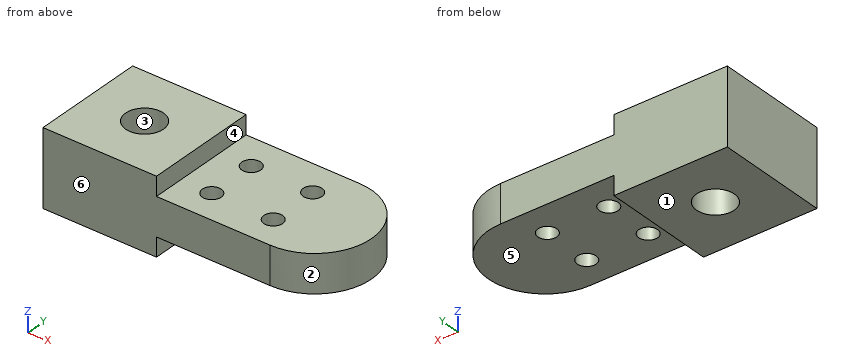
from build123d import *

# Parameters (mm, degrees)
F0_W     = 38.1
F0_H     = 38.1
F0_R     = 6.35
F0_R_2   = 3.175
F1_DEPTH = 25.4
F2_W     = 38.1
F2_H     = 6.35
F3_DEPTH = 38.101
F4_W     = 19.165852
F4_H     = 6.453032
F4_H_2   = 6.35
F5_DEPTH = 38.101


with BuildPart() as f1:
    # F0 (on Top) → F1 (new body)
    with BuildSketch(Plane.XY):
        with Locations((19.05, 19.05)):
            Rectangle(F0_W, F0_H)
        with Locations((19.05, 19.05)):
            Circle(F0_R, mode=Mode.SUBTRACT)
        with BuildLine():
            Line((38.1, 38.1), (38.1, 0))
            Line((38.1, 0), (76.2, 0))
            ThreePointArc((76.2, 0), (95.25, 19.05), (76.2, 38.1))
            Line((76.2, 38.1), (38.1, 38.1))
        make_face()
        with Locations((48.55017, 10.277208)):
            Circle(F0_R_2, mode=Mode.SUBTRACT)
        with Locations((69.168031, 10.277208)):
            Circle(F0_R_2, mode=Mode.SUBTRACT)
        with Locations((48.55017, 27.046405)):
            Circle(F0_R_2, mode=Mode.SUBTRACT)
        with Locations((69.168031, 27.046405)):
            Circle(F0_R_2, mode=Mode.SUBTRACT)
    extrude(amount=F1_DEPTH)

    # F2 (on face) → F3 (cut, through all)
    with BuildSketch(Plane.XZ):
        with Locations((57.15, 22.225)):
            Rectangle(F2_W, F2_H)
        with Locations((57.15, 3.175)):
            Rectangle(F2_W, F2_H)
    extrude(amount=-F3_DEPTH, mode=Mode.SUBTRACT)

    # F4 (on face) → F5 (cut, through all)
    with BuildSketch(Plane.XZ):
        with Locations((85.782926, 22.276516)):
            Rectangle(F4_W, F4_H)
        with Locations((85.782926, 3.175)):
            Rectangle(F4_W, F4_H_2)
    extrude(amount=-F5_DEPTH, mode=Mode.SUBTRACT)


solid = f1.part
The model under review builds one solid part; all positions refer to its coordinate system, in mm. Face numbers are marked on the shaded views. A direction names the side the tool comes from. Round coordinates to 2 decimals unless told otherwise and drop trailing zeros. Write each loop counter-clockwise with the first axis right and the second up, starting at its lowest first coordinate (ties: lowest second). Pieces come first, ordered by that corner, then holes. Notation, with made-up numbers: M 20.5,84 L 66.5,84 A26 ccw 66.5,117 Z; hole C -29,42 d7. An arc over 180 degrees is marked long. Answer as CSV lines item,"result". Start each with the question number.
Q1. Consider section A-A, the plane x = 19.05. Give the boundary of the cut face in (y, z).
Q2. The part is to be moulded in two halves that separate along X. For the marked faces 1, 2 and 3, say which applies: +X half, -X half, draft (parallel to the pull), parting line (faces both ways), or undercut.
Q3. Consider section C-C, the plane x = 67. Give the boundary of the cut face in (y, z), then the cut area to 3 significant figures.
Q4. Tool access review of the marked faces 4, 5 and 6: name each direction out of +Z, -Z, +X, -X, +Y, -Y from which nothing blocks a thin tool from reaching the whole face with its end or side.
Q5. Consider section D-D, the plane z = 11.5. Give the boundary of the cut face in (x, y) (3 decimals).
Q6. Clearance check with flat-ended pins moving along their axes: P1, Ø7.5, axis at x = 19.05, y = 19.05, coming from the -Z side; P2, Ø5, axis at x = 41.5, y = 23.5, coming from the -Z side; P3, Ø3, axis at y = 10.5, z = 3, coming from the +X side; P4, Ø4, axis at x = 79.5, y = 22, coming from the +Z side. State where each tip first meets the part, or that it passes through.
Q7. Wall thickness on line 1 along Y through (x, z) = (19.05, 9.75); line 2 along X through (y, z) = (19, 7); line 3 along Z through (x, y) = (72.5, 10.5): over which ranges is each line inside the solid? List them lowest first.
Q8. Consider section B-B, the plane y = 19.05. Give the boundary of the cut face in (x, z), then the cut area to 3 significant figures.
Result set:
1,outline,"M 0,0 L 12.7,0 L 12.7,25.4 L 0,25.4 Z; M 25.4,0 L 38.1,0 L 38.1,25.4 L 25.4,25.4 Z"
2,face 1,"draft"
2,face 2,"+X half"
2,face 3,"undercut"
3,outline,"M 0,6.35 L 7.96,6.35 L 7.96,19.05 L 0,19.05 Z; M 12.6,6.35 L 24.73,6.35 L 24.73,19.05 L 12.6,19.05 Z; M 29.37,6.35 L 38.1,6.35 L 38.1,19.05 L 29.37,19.05 Z"
3,area,"366 mm²"
4,face 4,"+Z, +X, +Y, -Y"
4,face 5,"-Z, +X, +Y, -Y"
4,face 6,"+Z, -Z, +X, -X, -Y"
5,outline,"M 0,0 L 76.2,0 A19.05 ccw 76.2,38.1 L 0,38.1 Z; hole C 19.05,19.05 d12.7; hole C 48.55,10.277 d6.35; hole C 48.55,27.046 d6.35; hole C 69.168,10.277 d6.35; hole C 69.168,27.046 d6.35"
6,P1,"passes through"
6,P2,"stops at z = 6.35"
6,P3,"stops at x = 38.1"
6,P4,"stops at z = 19.05"
7,line 1,"y = 0 to 12.7, 25.4 to 38.1"
7,line 2,"x = 0 to 12.7, 25.4 to 95.25"
7,line 3,"z = 6.35 to 19.05"
8,outline,"M 0,0 L 12.7,0 L 12.7,25.4 L 0,25.4 Z; M 25.4,0 L 38.1,0 L 38.1,6.35 L 95.25,6.35 L 95.25,19.05 L 38.1,19.05 L 38.1,25.4 L 25.4,25.4 Z"
8,area,"1,370 mm²"
